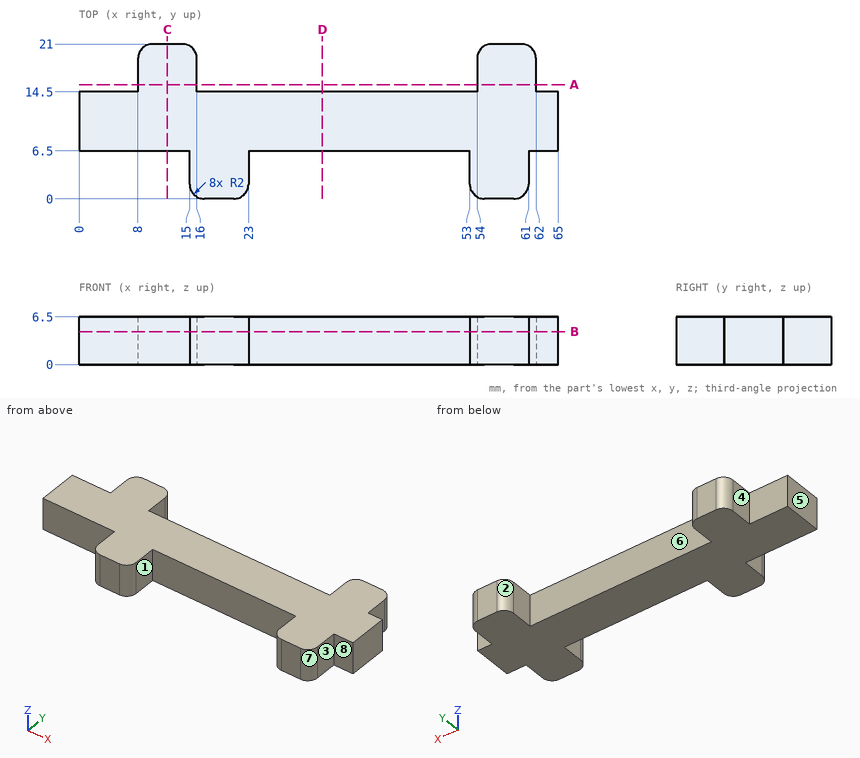
Check sheet for the drawn part. Datum: minimum x, y, z corner. Units: mm. A direction names the side the tool comes from. Give positions to 0.01 mm unless a question says otherwise; leave off trailing zeros. Order: outer loops, then holes, each group sorted by start corner. A loop starts at its lowest first (then second) coordinate and runs counter-clockwise, first axis right, second up. Notation, with made-up numbers: (49, -36.5) -> (106, -36.5) arc R24 cw to (106, -4.5) -> close; hole circle Ø5 at (39.5, -37). An arc over 180 degrees is marked (long way). One line per item, written item: value.
(1) Sectioned sample at D-D on x = 33. Record the cut outline in (y, z), then the cut area to 3 significant figures.
Final values:
outline: (6.5, 0) -> (14.5, 0) -> (14.5, 6.5) -> (6.5, 6.5) -> close
area: 52.0 mm^2
(2) Sectioned sample at A-A on y = 15.5. Record the cut outline in (x, z), then the cut area to 3 significant figures.
Final values:
outline: (8, 0) -> (16, 0) -> (16, 6.5) -> (8, 6.5) -> close; (54, 0) -> (62, 0) -> (62, 6.5) -> (54, 6.5) -> close
area: 104 mm^2
(3) Draft check along X on the marked faces 5, 6, 7 and 8. Enter one of: pulls with the +X half, pulls with the -X half, needs draft (parallel to the pull), parting line crosses it, or undercut.
Final values:
face 5: pulls with the -X half
face 6: undercut
face 7: pulls with the +X half
face 8: needs draft
(4) Tool access check on the marked faces 1, 2, 3 and 4. Record the directions out of +Z, -Z, +X, -X, +Y, -Y that give a thin tool (end or side, any length) a straight path to the whole face; none if there is none.
Final values:
face 1: +Z, -Z, -Y
face 2: +Z, -Z, +Y
face 3: +Z, -Z, +X, -Y
face 4: +Z, -Z, -X, +Y
(5) Gauge pin test, flat ends, axial feed: pin 1 (1.3 mm diameter, centred on y = 5.5, z = 5, fed in from +X); pin 2 (2 mm diameter, centred on y = 16, z = 4.5, fed in from +X); pin 3 (2 mm diameter, centred on x = 18, y = 18, fed in from +Z); pin 4 (2 mm diameter, centred on y = 17.5, z = 4.5, fed in from -X). Record the tip position at first contact, or that the pin passes through.
Final values:
pin 1: x = 61
pin 2: x = 62
pin 3: through
pin 4: x = 8
(6) Sectioned sample at C-C on x = 12. Record the cut outline in (y, z), then the cut area to 4 significant figures.
Final values:
outline: (6.5, 0) -> (21, 0) -> (21, 6.5) -> (6.5, 6.5) -> close
area: 94.25 mm^2
(7) Sectioned sample at B-B on z = 4.5. Record the cut outline in (x, y).
Final values:
outline: (0, 6.5) -> (15, 6.5) -> (15, 2) arc R2 ccw to (17, 0) -> (21, 0) arc R2 ccw to (23, 2) -> (23, 6.5) -> (53, 6.5) -> (53, 2) arc R2 ccw to (55, 0) -> (59, 0) arc R2 ccw to (61, 2) -> (61, 6.5) -> (65, 6.5) -> (65, 14.5) -> (62, 14.5) -> (62, 19) arc R2 ccw to (60, 21) -> (56, 21) arc R2 ccw to (54, 19) -> (54, 14.5) -> (16, 14.5) -> (16, 19) arc R2 ccw to (14, 21) -> (10, 21) arc R2 ccw to (8, 19) -> (8, 14.5) -> (0, 14.5) -> close
(8) Scan lines: line 1 along X through (y, z) = (16.25, 5); line 2 along X through (y, z) = (2, 4.75); line 3 along Y through (x, z) = (4.5, 2). Record each from-to range of solid material in increasing order. Write a range as [from, to].
Final values:
line 1: [8, 16], [54, 62]
line 2: [15, 23], [53, 61]
line 3: [6.5, 14.5]
